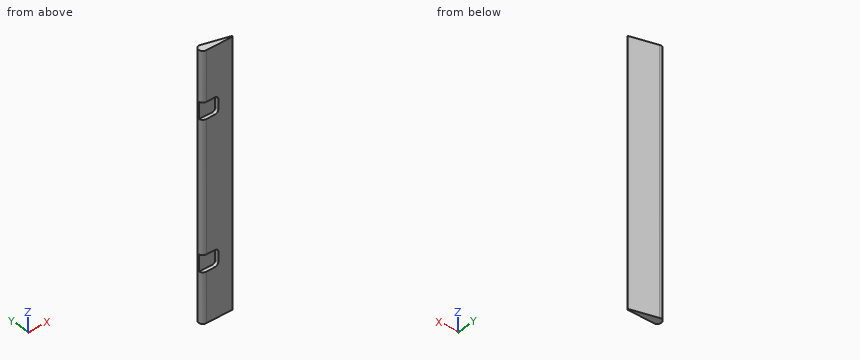
from build123d import *

# Parameters (mm, degrees)
BOSS_EXTRUDE1_DEPTH = 238
SKETCH3_W           = 15
SKETCH3_H           = 15
CUT_EXTRUDE1_DEPTH  = 54
FILLET1_R           = 0.5
FILLET2_R           = 3


with BuildPart() as part:
    # Sketch2 → Boss-Extrude1 (new body)
    with BuildSketch(Plane.XY.offset(-3)):
        with BuildLine():
            Line((446.391965645, 20.11245238), (474.43313548, 20.11245238))
            Line((474.43313548, 20.11245238), (447.390900992, 27.530319971))
            ThreePointArc((447.390900992, 27.530319971), (442.649552271, 24.39262378), (446.391965645, 20.11245238))
        make_face()
    extrude(amount=BOSS_EXTRUDE1_DEPTH)

    # Sketch3 → Cut-Extrude1 (cut)
    with BuildSketch(Plane.XZ.offset(30.589717262)):
        with Locations((450.115770482, 182.5)):
            Rectangle(SKETCH3_W, SKETCH3_H)
        with Locations((450.115770482, 49.5)):
            Rectangle(SKETCH3_W, SKETCH3_H)
    extrude(amount=-CUT_EXTRUDE1_DEPTH, mode=Mode.SUBTRACT)

    # Fillet1
    fillet1_edges = [part.edges().sort_by_distance(p)[0] for p in [
        (474.43313548, 20.11245238, 116),
    ]]
    fillet(fillet1_edges, radius=FILLET1_R)

    # Fillet2
    fillet2_edges = [part.edges().sort_by_distance(p)[0] for p in [
        (457.615770482, 21.761367559, 190),
        (457.615770482, 21.761367559, 175),
        (457.615770482, 21.761367559, 57),
        (457.615770482, 21.761367559, 42),
    ]]
    fillet(fillet2_edges, radius=FILLET2_R)


solid = part.part
Here's how the part is built. I have some questions about the finished solid (model axes, mm). Coordinates: 2 decimals unless noted, no trailing zeros. Loops run counter-clockwise (first coordinate to the right, second up) from the corner with the lowest first, then second, coordinate; pieces in that order, holes last.
1. I need wall thicknesses on L1, parallel to Z at x = 451, y = 23; L2, parallel to Z at x = 456.75, y = 23; L3, parallel to Y at x = 445.5, z = 118. Which ranges of each line are inside material? Lowest first, please.
2. Imagine slicing it at A-A, the plane z = 142. Please give me the cut outline in (x, y), and give its area (3 significant figures).
3. For P1, Ø4.5, axis at x = 451, z = 186, coming from the -Y side; P2, Ø3, axis at y = 23.5, z = 85.5, coming from the -X side, each with a flat end and sliding along its axis, tell me the tip position at first contact or that it passes through.
4. Imagine slicing it at B-B, the plane x = 464.5. Please give me the cut outline in (y, z), and give its area (3 significant figures).
Taken from the geometry:
1. L1: z = -3 to 42, 57 to 175, 190 to 235
1. L2: z = -3 to 42.89, 56.11 to 175.89, 189.11 to 235
1. L3: y = 20.22 to 27.56
2. outline: (446.39, 20.11) - (470.72, 20.11) arc R0.5 ccw to (470.85, 21.09) - (447.39, 27.53) arc R3.78 ccw (long way) to start
2. area: 129 mm2
3. P1: stops at y = 23.41
3. P2: stops at x = 442.62
4. outline: (20.11, -3) - (22.84, -3) - (22.84, 235) - (20.11, 235) - close
4. area: 648 mm2
